Input: dimensioned drawing with shaded views. Units: mm. Origin: part minimum x, y, z. Give positions to 0.01 mm unless a question says otherwise; leave off trailing zeros. Write each loop counter-clockwise with the first axis right and the second up, starting at its lowest first coordinate (ties: lowest second). Pieces come first, ordered by that corner, then holes.
Q1. Section A-A (z = 3.5). Return the cut outline in (x, y).
Q2. Pin query (flat end, axial travel): pin 1 Ø2 at (y, z) = (1.5, 7) entering from -X. Return the tip coordinate at first contact, or that it passes through.
Q3. Section C-C (z = 15). Return the cut outline in (x, y), plus the area to 3 significant figures.
Q4. Line query: line 1 (Z direction, x = 17.5, y = 2.7); line 2 (X direction, y = 2.9, z = 8.5); line 3 (X direction, y = 4.35, z = 15). Output: solid intervals per line, ascending.
Q5. Mould query, pull axis X, two halves, no side actions, for the marked faces 1, 2 and 3. Classes: +X half, -X half, draft (parallel to the pull), parting line (faces both ways), or undercut.
Q6. Section D-D (x = 17.5). Return the cut outline in (y, z).
Q7. Section B-B (x = 3.5). Return the cut outline in (y, z).
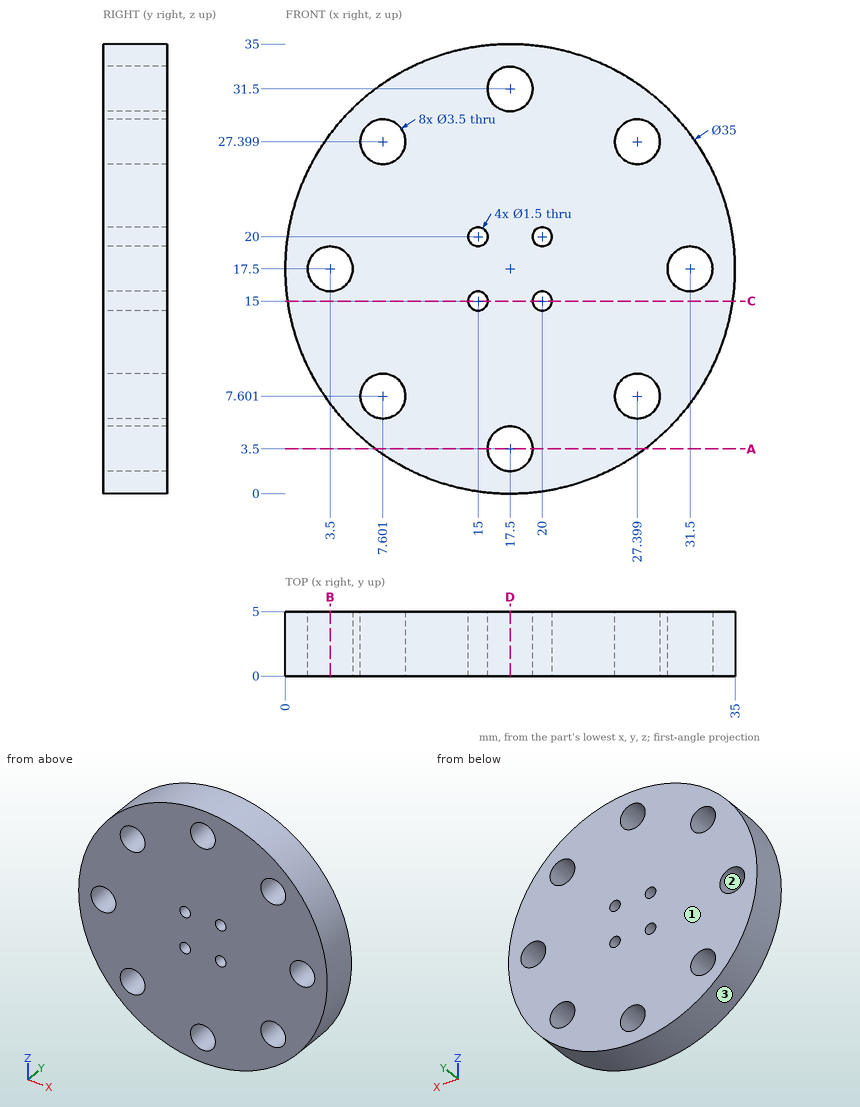
Computed:
1. outline: (7, 0) - (15.75, 0) - (15.75, 5) - (7, 5) - close; (19.25, 0) - (28, 0) - (28, 5) - (19.25, 5) - close
2. pin 1: stops at x = 2.8
3. outline: (0.18, 0) - (14.25, 0) - (14.25, 5) - (0.18, 5) - close; (15.75, 0) - (19.25, 0) - (19.25, 5) - (15.75, 5) - close; (20.75, 0) - (34.82, 0) - (34.82, 5) - (20.75, 5) - close
3. area: 158 mm2
4. line 1: z = 0 to 1.75, 5.25 to 29.75, 33.25 to 35
4. line 2: x = 2.49 to 6.1, 9.1 to 25.9, 28.9 to 32.51
4. line 3: x = 0.18 to 14.25, 15.75 to 19.25, 20.75 to 34.82
5. face 1: draft
5. face 2: undercut
5. face 3: parting line
6. outline: (0, 0) - (5, 0) - (5, 1.75) - (0, 1.75) - close; (0, 5.25) - (5, 5.25) - (5, 29.75) - (0, 29.75) - close; (0, 33.25) - (5, 33.25) - (5, 35) - (0, 35) - close
7. outline: (0, 7) - (5, 7) - (5, 15.75) - (0, 15.75) - close; (0, 19.25) - (5, 19.25) - (5, 28) - (0, 28) - close
